Part model, mm, in its own coordinate system. Give positions to 0.01 mm unless a question says otherwise; leave off trailing zeros. Order: outer loops, then holes, each group sorted by start corner. A loop starts at its lowest first (then second) coordinate and runs counter-clockwise, first axis right, second up. Notation, with made-up numbers: M 2,23 L 26,23 A20 ccw 26,42 Z; hole C 57.25,21 d7. An arc over 180 degrees is marked long. Answer as a JSON object with one key per item and string values.
from build123d import *

# Parameters (mm, degrees)
SKETCH_2_R          = 3
EXTRUDE_1_DEPTH     = 540
SKETCH_3_R          = 2
EXTRUDE_2_DEPTH     = 9.5
SKETCH_4_R          = 3
EXTRUDE_3_DEPTH     = 20
SKETCH_6_W          = 1
SKETCH_6_H          = 10
CUT_EXTRUDE_2_DEPTH = 5
SKETCH_7_R          = 2
CUT_EXTRUDE_3_DEPTH = 10


with BuildPart() as part:
    # 草图2 → 凸台-拉伸1 (new body)
    with BuildSketch(Plane(origin=(0, 0, 0), x_dir=(1, 0, 0), z_dir=(0, 1, 0))):
        with Locations(Location((0, 0, 0), (0, 0, 270))):
            Circle(SKETCH_2_R)
    extrude(amount=EXTRUDE_1_DEPTH)

    # 草图3 → 凸台-拉伸2 (add)
    with BuildSketch(Plane.XZ):
        with Locations(Location((0, 0, 0), (0, 0, 90))):
            Circle(SKETCH_3_R)
    extrude(amount=EXTRUDE_2_DEPTH)

    # 草图4 → 凸台-拉伸3 (add)
    with BuildSketch(Plane(origin=(0, 540, 0), x_dir=(1, 0, 0), z_dir=(0, 1, 0))):
        with Locations(Location((0, 0, 0), (0, 0, 270))):
            Circle(SKETCH_4_R)
    extrude(amount=EXTRUDE_3_DEPTH)

    # 草图6 → 切除-拉伸2 (cut, symmetric)
    with BuildSketch(Plane.XY):
        with Locations((-2.5, 550)):
            Rectangle(SKETCH_6_W, SKETCH_6_H)
        with Locations((2.5, 550)):
            Rectangle(SKETCH_6_W, SKETCH_6_H)
    extrude(amount=CUT_EXTRUDE_2_DEPTH, both=True, mode=Mode.SUBTRACT)

    # 草图7 → 切除-拉伸3 (cut)
    with BuildSketch(Plane.ZY.offset(2)):
        with Locations((0, 550)):
            Circle(SKETCH_7_R)
    extrude(amount=-CUT_EXTRUDE_3_DEPTH, mode=Mode.SUBTRACT)


solid = part.part
1. Cut at B-B on y = 166. Give the cut face in (x, z), plus the area to 3 significant figures.
Worked answers:
{"outline": "C 0,0 d6", "area": "28.3 mm^2"}
2. Cut at A-A on z = 0. Give the cut face in (x, y), plus the area to 3 significant figures.
Worked answers:
{"outline": "M -3,0 L -2,0 L -2,-9.5 L 2,-9.5 L 2,0 L 3,0 L 3,545 L 2,545 L 2,548 L -2,548 L -2,545 L -3,545 Z; M -3,555 L -2,555 L -2,552 L 2,552 L 2,555 L 3,555 L 3,560 L -3,560 Z", "area": "3,360 mm^2"}
3. Pin check, flat tips, straight feed: P1, Ø0.8, axis at x = 2.5, z = -0.5, coming from the -Y side; P2, Ø3.5, axis at y = 551, z = 0.5, coming from the -X side; P3, Ø2, axis at y = 548.5, z = -0.5, coming from the +X side. Stop position of each tip, or through.
Worked answers:
{"P1": "stops at y = 0", "P2": "stops at x = -2", "P3": "stops at x = 2"}
4. Probe line 1 along Y through (x, z) = (0.95, 0); line 2 along Y through (x, z) = (1.55, 0.55); line 3 along Z through (x, y) = (0.2, 550). List the from-to ranges inside material, lowest first.
Worked answers:
{"line 1": "y = -9.5 to 548, 552 to 560", "line 2": "y = -9.5 to 548.08, 551.92 to 560", "line 3": "z = -2.99 to -2, 2 to 2.99"}
